from build123d import *

# Parameters (mm, degrees)
F0_R     = 5.588
F1_DEPTH = 1.905
F2_W     = 6.985
F2_H     = 6.985
F3_DEPTH = 1.905
F4_R     = 1.1303
F5_DEPTH = 3.81
F6_SIZE  = 0.508


with BuildPart() as f1:
    # F0 (on Top) → F1 (new body)
    with BuildSketch(Plane.XY):
        Circle(F0_R)
    extrude(amount=F1_DEPTH)

    # F2 (on face) → F3 (join)
    with BuildSketch(Plane.XY.offset(1.905)):
        Rectangle(F2_W, F2_H)
    extrude(amount=F3_DEPTH)

    # F4 (on face) → F5 (cut, through all)
    with BuildSketch(Plane.XY.offset(3.81)):
        Circle(F4_R)
    extrude(amount=-F5_DEPTH, mode=Mode.SUBTRACT)

    # F6
    f6_edges = [f1.edges().sort_by_distance(p)[0] for p in [
        (1.1303, 0, 1.905),
        (-1.1303, 0, 3.81),
        (-1.1303, 0, 0),
    ]]
    chamfer(f6_edges, length=F6_SIZE)


solid = f1.part
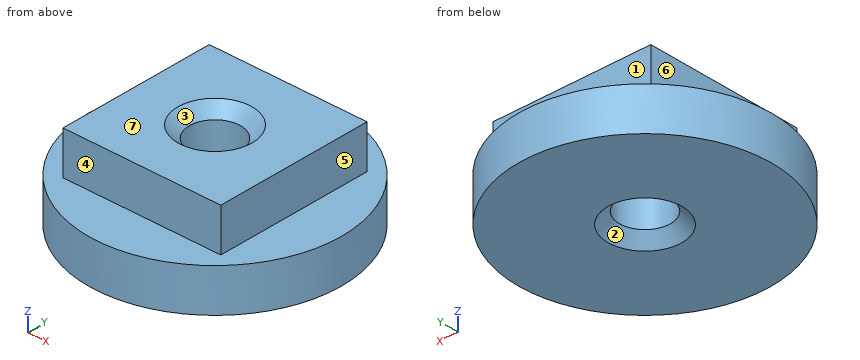
Check sheet for the modelled part. Datum: model origin and axes. Units: mm. Face numbers are marked on the shaded views. A direction names the side the tool comes from. Round coordinates to 2 decimals unless told otherwise and drop trailing zeros. Loops run counter-clockwise (first coordinate to the right, second up) from the corner with the lowest first, then second, coordinate; pieces in that order, holes last. Notation, with made-up numbers: (61, -30) -> (86, -30) arc R20 cw to (86, 0) -> close; hole circle Ø6 at (63.25, 23). An arc over 180 degrees is marked (long way). Put each result on its own line as item: value. Start each with the question number.
1. Section check C-C (z = 3.1). Enter the section's corners in (x, y), plus the area to 3 significant figures.
2. Section check A-A (y = 0). Enter the section's corners in (x, z) (1 decimal).
3. Access from +Z, -Z, +X, -X, +Y, -Y to the whole of each face (thin tool, end or side, straight path). Record for the marked faces 5, 6 and 7.
4. Scan lines: probe 1 along Y at (x, z) = (0, 1.25); probe 2 along Y at (x, z) = (0, 2.25); probe 3 along Z at (x, y) = (1.75, 4.75) (3 decimals). Record each from-to range of solid material in increasing order.
5. Draft check along Y on the marked faces 1, 2, 3 and 4. Enter one of: +Y half, -Y half, draft (parallel to the pull), parting line (faces both ways), or undercut.
6. Section check D-D (y = -2). Enter the section's corners in (x, z) (1 decimal).
7. Gauge pin test, flat ends, axial feed: pin 1 (1 mm diameter, centred on y = 0.5, z = 3, fed in from -X); pin 2 (1 mm diameter, centred on y = 1.5, z = 3, fed in from +X); pin 3 (2 mm diameter, centred on x = -1.5, z = 2.5, fed in from +Y). Record the tip position at first contact, or that the pin passes through.
Findings:
1. outline: (-3.49, -3.49) -> (3.49, -3.49) -> (3.49, 3.49) -> (-3.49, 3.49) -> close; hole circle Ø2.26 at (0, 0)
1. area: 44.8 mm^2
2. outline: (-5.6, 0) -> (-1.6, 0) -> (-1.1, 0.5) -> (-1.1, 3.3) -> (-1.6, 3.8) -> (-3.5, 3.8) -> (-3.5, 1.9) -> (-5.6, 1.9) -> close; (1.1, 0.5) -> (1.6, 0) -> (5.6, 0) -> (5.6, 1.9) -> (3.5, 1.9) -> (3.5, 3.8) -> (1.6, 3.8) -> (1.1, 3.3) -> close
3. face 5: +Z, +X, +Y, -Y
3. face 6: +Z, -X, +Y, -Y
3. face 7: +Z, +X, -X, +Y, -Y
4. probe 1: y = -5.59 to -1.13, 1.13 to 5.59
4. probe 2: y = -3.49 to -1.13, 1.13 to 3.49
4. probe 3: z = 0 to 1.905
5. face 1: +Y half
5. face 2: undercut
5. face 3: undercut
5. face 4: -Y half
6. outline: (-5.2, 0) -> (5.2, 0) -> (5.2, 1.9) -> (3.5, 1.9) -> (3.5, 3.8) -> (-3.5, 3.8) -> (-3.5, 1.9) -> (-5.2, 1.9) -> close
7. pin 1: stops at x = -3.49
7. pin 2: stops at x = 3.49
7. pin 3: stops at y = 5.54
